from build123d import *

# Parameters (mm, degrees)
SKETCH1_W           = 11
SKETCH1_H           = 8
SKETCH1_R           = 2
BOSS_EXTRUDE1_DEPTH = 4.3
CUT_EXTRUDE1_DEPTH  = 9
SKETCH3_W           = 6.77
SKETCH3_H           = 8
SKETCH3_R           = 2
BOSS_EXTRUDE2_DEPTH = 1.8
FILLET1_R           = 4
FILLET2_R           = 1


with BuildPart() as part:
    # Sketch1 → Boss-Extrude1 (new body)
    with BuildSketch(Plane(origin=(0, 0, 0), x_dir=(1, 0, 0), z_dir=(0, 1, 0))):
        Rectangle(SKETCH1_W, SKETCH1_H)
        Circle(SKETCH1_R, mode=Mode.SUBTRACT)
    extrude(amount=BOSS_EXTRUDE1_DEPTH)

    # Sketch2 → Cut-Extrude1 (cut, through all)
    with BuildSketch(Plane.XY.offset(4)):
        Polygon((-5.5, 2.66), (-2.84, 0), (-5.5, 0), align=None)
        Polygon((5.5, 2.66), (5.5, 0), (2.84, 0), align=None)
    extrude(amount=-CUT_EXTRUDE1_DEPTH, mode=Mode.SUBTRACT)

    # Sketch3 → Boss-Extrude2 (add)
    with BuildSketch(Plane(origin=(0, 4.3, 0), x_dir=(1, 0, 0), z_dir=(0, 1, 0))):
        Rectangle(SKETCH3_W, SKETCH3_H)
        Circle(SKETCH3_R, mode=Mode.SUBTRACT)
    extrude(amount=BOSS_EXTRUDE2_DEPTH)

    # Fillet1
    fillet1_edges = [part.edges().sort_by_distance(p)[0] for p in [
        (3.385, 5.2, -4),
        (-3.385, 5.2, 4),
    ]]
    fillet(fillet1_edges, radius=FILLET1_R)

    # Fillet2
    fillet2_edges = [part.edges().sort_by_distance(p)[0] for p in [
        (5.5, 3.48, 4),
        (-5.5, 3.48, -4),
    ]]
    fillet(fillet2_edges, radius=FILLET2_R)


solid = part.part
Geometry check sheet. Reference: the model listing, model coordinates, mm. A direction names the side the tool comes from. Give positions to 0.01 mm unless a question says otherwise; leave off trailing zeros. Loops run counter-clockwise (first coordinate to the right, second up) from the corner with the lowest first, then second, coordinate; pieces in that order, holes last. Notation, with made-up numbers: (6.25, -6) -> (40.25, -6) arc R13 ccw to (40.25, 18) -> close; hole circle Ø5 at (58, -8). An arc over 180 degrees is marked (long way). Answer in a Markdown table with one row per item. Add a question column.
1) Cross-section at C-C on z = 1.25. Record the boundary of the cut face in (x, y) (3 decimals).
2) Cross-section at A-A on y = 3. Record the boundary of the cut face in (x, z).
3) Gauge pin test, flat ends, axial feed: P1, Ø1, axis at x = 1.5, y = 5, coming from the -Z side; P2, Ø0.9, axis at y = 5.5, z = -2, coming from the -X side (3 decimals); P3, Ø3.5, axis at x = 0, z = 0, coming from the +Y side. Record the tip position at first contact, or that the pin passes through.
4) Material ranges on probe 1 along Z at (x, y) = (0, 2); probe 2 along X at (y, z) = (3.5, 0); probe 3 along X at (y, z) = (1.5, 0), recorded low to high. Write a range as from..to.
5) Set-up check for faces 1 (the face through (-5, 4.3, 1)), 2 (the face through (4, 4.3, -1)), 3 (the face through (-3.385, 5, -2)): record each of +Z, -Z, +X, -X, +Y, -Y from which the full face is reachable in a straight line by a thin tool's end or side.
6) Draft check along Z on faces 4 (the face through (-1, 2, 4)), 5 (the face through (0, 3, 2)), 6 (the face through (4.15, 1.31, 0.06)), 7 (the face through (2.24, 5.21, -2.8)). Enter one of: pulls with the +Z half, pulls with the -Z half, needs draft (parallel to the pull), parting line crosses it, or undercut.
7) Cross-section at D-D on z = 2.25. Record the boundary of the cut face in (x, y) (3 decimals), and give its area (3 significant figures).
8) Cross-section at B-B on x = 1.5. Record the boundary of the cut face in (y, z).
Outcome:
| question | item | result |
|---|---|---|
| 1 | outline | (-5.5, 2.66) -> (-2.84, 0) -> (-1.561, 0) -> (-1.561, 6.1) -> (-3.185, 6.1) -> (-3.185, 4.3) -> (-5.5, 4.3) -> close; (1.561, 0) -> (2.84, 0) -> (5.5, 2.66) -> (5.5, 4.3) -> (3.385, 4.3) -> (3.385, 6.1) -> (1.561, 6.1) -> close |
| 2 | outline | (-5.5, -3) arc R1 ccw to (-4.5, -4) -> (5.5, -4) -> (5.5, 3) arc R1 ccw to (4.5, 4) -> (-5.5, 4) -> close; hole circle Ø4 at (0, 0) |
| 3 | P1 | stops at z = -3.66 |
| 3 | P2 | stops at x = -3.385 |
| 3 | P3 | passes through |
| 4 | probe 1 | z = -4..-2, 2..4 |
| 4 | probe 2 | x = -5.5..-2, 2..5.5 |
| 4 | probe 3 | x = -4.34..-2, 2..4.34 |
| 5 | face 1 | +Z, -X, +Y |
| 5 | face 2 | -Z, +X, +Y |
| 5 | face 3 | +Z, -Z, -X, +Y |
| 6 | face 4 | pulls with the +Z half |
| 6 | face 5 | undercut |
| 6 | face 6 | needs draft |
| 6 | face 7 | pulls with the -Z half |
| 7 | outline | (-5.5, 2.66) -> (-2.84, 0) -> (2.84, 0) -> (5.5, 2.66) -> (5.5, 4.3) -> (3.385, 4.3) -> (3.385, 6.1) -> (-2.692, 6.1) -> (-2.692, 4.3) -> (-5.5, 4.3) -> close |
| 7 | area | 51.2 mm^2 |
| 8 | outline | (0, -4) -> (4.3, -4) -> (4.3, -3.4) -> (6.1, -3.4) -> (6.1, -1.32) -> (0, -1.32) -> close; (0, 1.32) -> (6.1, 1.32) -> (6.1, 4) -> (0, 4) -> close |
